Geometry: final body of the model. Coordinates: model frame, mm. A direction names the side the tool comes from. Coordinates: 2 decimals unless noted, no trailing zeros. Order: outer loops, then holes, each group sorted by start corner. A loop starts at its lowest first (then second) coordinate and runs counter-clockwise, first axis right, second up. Notation, with made-up numbers: M -28,65.5 L 17,65.5 A11 cw 17,73.5 Z; hole C 43.25,29 d11. An arc over 180 degrees is marked long. Use CSV: the item, a comma, the result in double quotes. Start each with the question number.
Q1. Section query C-C, the plane z = 86. Output: boundary loops of the cut face in (x, y).
Q2. Ray query, probe 1 along Z at (x, y) = (30, 35.25) (3 decimals); probe 2 along Z at (x, y) = (-14, -3); probe 3 along Y at (x, z) = (5, 49.5). Return the intervals inside material, ascending.
Q3. Section query A-A, the plane z = 55. Output: boundary loops of the cut face in (x, y) (3 decimals).
Q4. Section query B-B, the plane x = 14.5. Output: boundary loops of the cut face in (y, z), and give its area (3 significant figures).
Q5. Mould query, pull axis X, two halves, no side actions, for faces 4 (the face through (1, 18.07, 55)), 5 (the face through (44.04, 0.94, 84.49)), 6 (the face through (-31, 25.07, 52)). Classes: +X half, -X half, draft (parallel to the pull), parting line (faces both ways), or undercut.
Q6. Access query for faces 1 (the face through (-32.51, 21.52, 59.44)), 2 (the face through (2.76, -8.61, 37.43)), 3 (the face through (44.04, 0.94, 25.03)). Directions: +Z, -Z, +X, -X, +Y, -Y. A direction counts if a zero-diameter tool reaches every point of the face in a straight line with its end or side. Return the directions, or none.
Q7. First-contact query: P1, Ø6, axis at x = 30, z = 55, coming from the -Y side; P2, Ø4, axis at x = 24.5, z = 52.5, coming from the -Y side; P3, Ø4, axis at x = 30.5, y = 1, coming from the +Z side; P4, Ø1.5, axis at y = -3, z = 43, coming from the -X side. Flat tips, straight axial feed; report the tip coordinate or a pass-through.
from build123d import *

# Parameters (mm, degrees)
F1_DEPTH  = 110
F3_W      = 92
F3_H      = 25
F4_DEPTH  = 80
F5_SIZE2  = 10
F5_SIZE   = 50
F6_SIZE2  = 10
F6_SIZE   = 50
F7_SIZE2  = 10
F7_SIZE   = 35
F8_SIZE2  = 10
F8_SIZE   = 35
F9_SIZE2  = 5
F9_SIZE   = 35
F10_SIZE2 = 5
F10_SIZE  = 30
F11_R     = 10
F12_R     = 5
F14_D     = 5.25
F16_DEPTH = 7


with BuildPart() as f1:
    # F0 (on Top) → F1 (new body)
    with BuildSketch(Plane.XY):
        Polygon((46, 43.0696749699), (-46, 43.0696749699), (-46, -32.9303250301), (46, -19.9303250301), align=None)
    extrude(amount=F1_DEPTH)

    # F3 (on offset) → F4 (cut)
    with BuildSketch(Plane(origin=(0, 18.0696749699, 0), x_dir=(-1, 0, 0), z_dir=(0, 1, 0))):
        with Locations((0, 55)):
            Rectangle(F3_W, F3_H)
    extrude(amount=-F4_DEPTH, mode=Mode.SUBTRACT)

    # F5
    f5_edges = [f1.edges().sort_by_distance(p)[0] for p in [
        (0, -26.430325, 110),
    ]]
    f5_side = f1.faces().sort_by_distance((-1.434053, 8.218356, 110))[0]
    chamfer(f5_edges, length=F5_SIZE, length2=F5_SIZE2, reference=f5_side)

    # F6
    f6_edges = [f1.edges().sort_by_distance(p)[0] for p in [
        (0, -26.430325, 0),
    ]]
    f6_side = f1.faces().sort_by_distance((-1.434053, 8.218356, 0))[0]
    chamfer(f6_edges, length=F6_SIZE, length2=F6_SIZE2, reference=f6_side)

    # F7
    f7_edges = [f1.edges().sort_by_distance(p)[0] for p in [
        (0, -26.430325, 67.5),
    ]]
    f7_side = f1.faces().sort_by_distance((-2.2397, -4.338565, 67.5))[0]
    chamfer(f7_edges, length=F7_SIZE, length2=F7_SIZE2, reference=f7_side)

    # F8
    f8_edges = [f1.edges().sort_by_distance(p)[0] for p in [
        (0, -26.430325, 42.5),
    ]]
    f8_side = f1.faces().sort_by_distance((-2.2397, -4.338565, 42.5))[0]
    chamfer(f8_edges, length=F8_SIZE, length2=F8_SIZE2, reference=f8_side)

    # F9
    f9_edges = [f1.edges().sort_by_distance(p)[0] for p in [
        (46, -19.930325, 21.25),
        (46, -19.930325, 88.75),
    ]]
    f9_side = f1.faces().sort_by_distance((46, 16.743522, 41.232364))[0]
    chamfer(f9_edges, length=F9_SIZE, length2=F9_SIZE2, reference=f9_side)

    # F10
    f10_edges = [f1.edges().sort_by_distance(p)[0] for p in [
        (-46, -32.930325, 88.75),
        (-46, -32.930325, 21.25),
    ]]
    f10_side = f1.faces().sort_by_distance((-46, 10.243522, 41.162988))[0]
    chamfer(f10_edges, length=F10_SIZE, length2=F10_SIZE2, reference=f10_side)

    # F11
    f11_edges = [f1.edges().sort_by_distance(p)[0] for p in [
        (-46, 30.318028, 110),
        (-46, 30.318028, 0),
        (46, 36.818028, 0),
        (46, 36.818028, 110),
    ]]
    fillet(f11_edges, radius=F11_R)

    # F12
    f12_edges = [f1.edges().sort_by_distance(p)[0] for p in [
        (-42.964823, -20.893414, 7.701231),
        (42.845838, -7.674494, 7.484682),
        (42.845838, -7.674494, 102.515318),
        (-42.964823, -20.893414, 102.298769),
    ]]
    fillet(f12_edges, radius=F12_R)

    # F14 (through all)
    with Locations(Plane(origin=(0, 43.0696749699, 0), x_dir=(-1, 0, 0), z_dir=(0, 1, 0))):
        with Locations((-30, 55), (30, 55)):
            Hole(F14_D / 2)

    # F15 (on face) → F16 (cut)
    with BuildSketch(Plane.XZ.offset(-18.0696749699)):
        Polygon((-24.9, 52.0555136271), (-24.9, 57.9444863729), (-30, 60.8889727457), (-35.1, 57.9444863729), (-35.1, 52.0555136271), (-30, 49.1110272543), align=None)
        Polygon((24.9, 57.9444863729), (24.9, 52.0555136271), (30, 49.1110272543), (35.1, 52.0555136271), (35.1, 57.9444863729), (30, 60.8889727457), align=None)
    extrude(amount=-F16_DEPTH, mode=Mode.SUBTRACT)


solid = f1.part
Responses:
1,outline,"M -46,-2.93 L -41.05,-32.23 L 41.05,-20.63 L 46,15.07 L 46,43.07 L -46,43.07 Z"
2,probe 1,"z = 0 to 52.375, 57.625 to 110"
2,probe 2,"z = 4.97 to 39.69, 70.31 to 105.03"
2,probe 3,"y = 18.07 to 43.07"
3,outline,"M -46,18.07 L -35.1,18.07 L -35.1,25.07 L -32.625,25.07 L -32.625,43.07 L -46,43.07 Z; M -27.375,25.07 L -24.9,25.07 L -24.9,18.07 L 24.9,18.07 L 24.9,25.07 L 27.375,25.07 L 27.375,43.07 L -27.375,43.07 Z; M 32.625,25.07 L 35.1,25.07 L 35.1,18.07 L 46,18.07 L 46,43.07 L 32.625,43.07 Z"
4,outline,"M -24.38,10 L 26.12,0 L 43.07,0 L 43.07,110 L 26.12,110 L -24.38,100 L -24.38,77.5 L 10.97,67.5 L 18.07,67.5 L 18.07,42.5 L 10.97,42.5 L -24.38,32.5 Z"
4,area,"5,500 mm²"
5,face 4,"draft"
5,face 5,"+X half"
5,face 6,"undercut"
6,face 1,"-Y"
6,face 2,"+X, -Y"
6,face 3,"+Z, -Z, +X, -Y"
7,P1,"stops at y = 25.07"
7,P2,"stops at y = 18.07"
7,P3,"stops at z = 104.98"
7,P4,"passes through"
